from build123d import *

# Parameters (mm, degrees)
F0_R     = 18
F1_DEPTH = 500
F2_R     = 25
F3_DEPTH = 30
F5_DEPTH = 30


with BuildPart() as f1:
    # F0 (on Right) → F1 (new body, symmetric)
    with BuildSketch(Plane.YZ):
        Circle(F0_R)
    extrude(amount=F1_DEPTH, both=True)

    # F2 (on face) → F3 (join)
    with BuildSketch(Plane(origin=(-500, 0, 0), x_dir=(0, -1, 0), z_dir=(-1, 0, 0))):
        Circle(F2_R)
    extrude(amount=F3_DEPTH)

    # F4 (on face) → F5 (join)
    with BuildSketch(Plane(origin=(-530, 0, 0), x_dir=(0, -1, 0), z_dir=(-1, 0, 0))):
        Polygon((-7.696053, -23.785936), (16.751199, -18.557945), (24.447252, 5.227991), (7.696053, 23.785936), (-16.751199, 18.557945), (-24.447252, -5.227991), align=None)
    extrude(amount=F5_DEPTH)


solid = f1.part
Could you check a few things on this model? Use its own coordinates, in mm. A direction names the side the tool comes from. Round coordinates to 2 decimals unless told otherwise and drop trailing zeros. Loops run counter-clockwise (first coordinate to the right, second up) from the corner with the lowest first, then second, coordinate; pieces in that order, holes last. Notation, with made-up numbers: (-9.5, 37) -> (-3.5, 37) arc R12 ccw to (-3.5, 52) -> close; hole circle Ø2 at (77.5, 13.5). An arc over 180 degrees is marked (long way). Use CSV: the item, a comma, the result in double quotes.
(1) Will these pins go through, and if not, where does the flat tip stop? pin 1 Ø5 at (x, z) = (-93, 4) entering from +Y; pin 2 Ø10 at (x, y) = (-447.5, 7.5) entering from -Z; pin 3 Ø4 at (x, z) = (272, -15.5) entering from -Y.
Return value:
pin 1,"stops at y = 17.94"
pin 2,"stops at z = -17.83"
pin 3,"stops at y = -11.91"
(2) If I drill on probe 1 along Y at (x, z) = (250, -2.5); probe 2 along X at (y, z) = (21, -13.5); probe 3 along Z at (x, y) = (141, 2), over which ranges is the centre line in solid material (lowest first)? Write a range as [from, to].
Return value:
probe 1,"y = [-17.83, 17.83]"
probe 2,"x = [-530, -500]"
probe 3,"z = [-17.89, 17.89]"
(3) For faces 1 (the flat face through (-544.8, 4.4, 21.2)), 2 (the cylindrical face through (7, -2.343, 17.847)), 3 (the flat face through (-530, 10, -22)), 4 (the flat face through (-530, -3.8, 23.2)), which set-ups out of +Z, -Z, +X, -X, +Y, -Y let a thin tool reach every point of the face, with its end or its side?
Return value:
face 1,"+Z, -X, +Y"
face 2,"+X"
face 3,"-Z, -X"
face 4,"+Z, -X"
(4) Suppose I cut it at A-A on y = 0. Write out the boundary of the cut face in (x, z).
Return value:
outline,"(-560, -22.14) -> (-530, -22.14) -> (-530, -25) -> (-500, -25) -> (-500, -18) -> (500, -18) -> (500, 18) -> (-500, 18) -> (-500, 25) -> (-530, 25) -> (-530, 22.14) -> (-560, 22.14) -> close"
(5) Suppose I cut it at B-B on x = 37.5. Write out the boundary of the cut face in (y, z), plus the area to 3 significant figures.
Return value:
outline,"circle Ø36 at (0, 0)"
area,"1,020 mm²"
